The model under review builds one solid part; all positions refer to its coordinate system, in mm. Coordinates: 2 decimals unless noted, no trailing zeros. Write each loop counter-clockwise with the first axis right and the second up, starting at its lowest first coordinate (ties: lowest second). Pieces come first, ordered by that corner, then holes. Notation, with made-up numbers: (-35, -1.5) -> (-22, -1.5) arc R25 cw to (-22, 30.5) -> close; hole circle Ø3 at (-2.75, -11.75). An arc over 180 degrees is marked (long way). Write each question's results on one line, items separated by ' | '.
```python
from build123d import *

# Parameters (mm, degrees)
PIPERING_R   = 0.8
PIPERING_R_2 = 0.4


with BuildPart() as part:
    # Pipe: sweep along a path in PipeSke
    with BuildLine() as pipe_path:  # in the path sketch's own coordinates; laid on its plane below (add() does not lay a ready-made edge on the line's plane)
        Line((-2, 0), (0, 0))
        add(Edge.make_bspline(
            [(0, 0), (4.619948081, 0), (6, 0.035966381), (6, 1.704499781)],
            knots=[0, 0, 0, 0, 1, 1, 1, 1], degree=3))
        Line((6, 1.704499781), (6, 21.704499781))
    # PipeRing → Pipe (sweep)
    with BuildSketch(Plane(origin=(0, 0, 0), x_dir=(0, 0, -1), z_dir=(1, 0, 0))):
        Circle(PIPERING_R)
        Circle(PIPERING_R_2, mode=Mode.SUBTRACT)
    sweep(path=Plane.XY * pipe_path.line)


solid = part.part
```
Q1. Add section A-A (y = 16). Write out the cut boundary in (x, z).
Solution:
outline: circle Ø1.6 at (6, 0); hole circle Ø0.8 at (6, 0)
Q2. For line 1 (X direction, y = 16, z = 0); line 2 (Y direction, x = 0.75, z = 0), list the stretches that pass through material, from the lowest coordinate up. Write a range as from..to.
Solution:
line 1: 5.2..5.6, 6.4..6.8 | line 2: -0.8..-0.4, 0.4..0.8
Q3. Draft analysis for pull direction X (two halves, no side actions). For faces 1 (the cylindrical face through (6.78, 11.84, 0.17)), 2 (the cylindrical face through (5.603, 11.844, 0.052)), 3 (the cylindrical face through (-0.99, -0.49, 0.63)), state which applies: pulls with the +X half, pulls with the -X half, needs draft (parallel to the pull), parting line crosses it, or undercut.
Solution:
face 1: parting line crosses it | face 2: undercut | face 3: needs draft
